Model file for the job. Use its own axes, mm. A direction names the side the tool comes from. Round coordinates to 2 decimals unless told otherwise and drop trailing zeros. Loops run counter-clockwise (first coordinate to the right, second up) from the corner with the lowest first, then second, coordinate; pieces in that order, holes last. Notation, with made-up numbers: M 40.5,-33.75 L 86.5,-33.75 A25 cw 86.5,3.25 Z; hole C 68,15 d5. An arc over 180 degrees is marked long. Use a Markdown table: item, result. Add a question column.
Item 1: Tool access for faces 1 (the flat face through (120, 300, -252)), 2 (the flat face through (120, 302.54, -252)), 3 (the cylindrical face through (103.313, 298.748, -38.394)): list every direction of +Z, -Z, +X, -X, +Y, -Y with a clear straight run to the whole face (end or side of a thin tool).
Item 2: Saw through at C-C on z = -101. Write the cut outline in (x, y), then the cut area to 3 significant figures.
Item 3: Saw through at A-A on y = 309. Write the cut outline in (x, z).
Item 4: Pin check, flat tips, straight feed: P1, Ø16.5, axis at x = 246, y = 314, coming from the -Z side; P2, Ø24.5, axis at x = 225.5, y = 320.5, coming from the +Z side; P3, Ø16.5, axis at y = 324.5, z = -182.5, coming from the +X side. Stop position of each tip, or through.
Item 5: Saw through at B-B on x = 30.5. Write the cut outline in (y, z).
Item 6: Saw through at D-D on z = -146. Write the cut outline in (x, y), then the cut area to 3 significant figures.
Item 7: Wall check: L1, parallel to Z at x = 194, y = 215; L2, parallel to X at y = 152, z = -27; L3, parallel to Y at x = 249.5, z = -224.5. Give the ranges that are in metal, low to high. Write a range as from..to.
Item 8: Two-plate mould, pull along X, no slides. Class faces 4 (the flat face through (148, 148, -300)), 5 (the flat face through (274.589, 316, -134)), 6 (the flat face through (148, 148, -297.46)): +X half, -X half, draft (parallel to the pull), parting line (faces both ways), or undercut.
```python
from build123d import *

# Parameters (mm, degrees)
SKETCH1_W           = 300
SKETCH1_H           = 300
BOSS_EXTRUDE1_DEPTH = 300
SHELL1_T            = -2.54
SKETCH2_W           = 300
SKETCH2_H           = 300
BOSS_EXTRUDE2_DEPTH = 2.54
SKETCH3_R           = 15.897271206
SKETCH3_R_2         = 16.201962057
SKETCH3_R_3         = 17.191821314
SKETCH3_R_4         = 17.661116969
CUT_EXTRUDE1_DEPTH  = 2.54
SKETCH4_R           = 22.06299853
SKETCH4_R_2         = 19.946075444
BOSS_EXTRUDE3_DEPTH = 2.54
SKETCH5_R           = 19.013382907
CUT_EXTRUDE2_DEPTH  = 2.54
SKETCH6_W           = 69.704124702
SKETCH6_H           = 204.3475123
SKETCH6_W_2         = 60.465312628
SKETCH6_H_2         = 192.466149128
BOSS_EXTRUDE4_DEPTH = 30.48
SKETCH7_W           = 69.704124702
SKETCH7_H           = 204.3475123
BOSS_EXTRUDE5_DEPTH = 2.54


with BuildPart() as part:
    # Sketch1 → Boss-Extrude1 (new body)
    with BuildSketch(Plane(origin=(0, 0, 0), x_dir=(1, 0, 0), z_dir=(0, 1, 0))):
        with Locations((150, 150)):
            Rectangle(SKETCH1_W, SKETCH1_H)
    extrude(amount=BOSS_EXTRUDE1_DEPTH)

    # Shell1
    shell1_openings = [part.faces().sort_by_distance(p)[0] for p in [
        (150, 300, -150),
    ]]
    offset(amount=SHELL1_T, openings=shell1_openings, kind=Kind.INTERSECTION)

    # Sketch2 → Boss-Extrude2 (add)
    with BuildSketch(Plane(origin=(0, 300, 0), x_dir=(1, 0, 0), z_dir=(0, 1, 0))):
        with Locations((150, 150)):
            Rectangle(SKETCH2_W, SKETCH2_H)
    extrude(amount=-BOSS_EXTRUDE2_DEPTH)

    # Sketch3 → Cut-Extrude1 (cut)
    with BuildSketch(Plane(origin=(0, 300, 0), x_dir=(1, 0, 0), z_dir=(0, 1, 0))):
        with Locations(Location((241.55793996, 57.94356866, 0), (0, 0, 270))):
            Circle(SKETCH3_R)
        with Locations(Location((241.55793996, 206.697112563, 0), (0, 0, 270))):
            Circle(SKETCH3_R_2)
        with Locations(Location((120.554438902, 251.95787292, 0), (0, 0, 270))):
            Circle(SKETCH3_R_3)
        with Locations(Location((120.554438902, 34.565752922, 0), (0, 0, 270))):
            Circle(SKETCH3_R_4)
    extrude(amount=-CUT_EXTRUDE1_DEPTH, mode=Mode.SUBTRACT)

    # Sketch4 → Boss-Extrude3 (add)
    with BuildSketch(Plane(origin=(0, 300, 0), x_dir=(1, 0, 0), z_dir=(0, 1, 0))):
        with Locations(Location((120.554438902, 251.95787292, 0), (0, 0, 90))):
            Circle(SKETCH4_R)
        with Locations(Location((241.55793996, 206.697112563, 0), (0, 0, 90))):
            Circle(SKETCH4_R_2)
    extrude(amount=BOSS_EXTRUDE3_DEPTH)

    # Sketch5 → Cut-Extrude2 (cut)
    with BuildSketch(Plane(origin=(0, 300, 0), x_dir=(1, 0, 0), z_dir=(0, 1, 0))):
        with Locations(Location((241.852973127, 150.869372117, 0), (0, 0, 270))):
            Circle(SKETCH5_R)
    extrude(amount=-CUT_EXTRUDE2_DEPTH, mode=Mode.SUBTRACT)

    # Sketch6 → Boss-Extrude4 (add)
    with BuildSketch(Plane(origin=(0, 300, 0), x_dir=(1, 0, 0), z_dir=(0, 1, 0))):
        with Locations((239.736552446, 135.332520717)):
            Rectangle(SKETCH6_W, SKETCH6_H)
        with Locations((239.510491416, 134.641215144)):
            Rectangle(SKETCH6_W_2, SKETCH6_H_2, mode=Mode.SUBTRACT)
    extrude(amount=BOSS_EXTRUDE4_DEPTH)

    # Sketch7 → Boss-Extrude5 (add)
    with BuildSketch(Plane(origin=(0, 330.48, 0), x_dir=(1, 0, 0), z_dir=(0, 1, 0))):
        with Locations((239.736552446, 135.332520717)):
            Rectangle(SKETCH7_W, SKETCH7_H)
    extrude(amount=BOSS_EXTRUDE5_DEPTH)


solid = part.part
```
Entries:
| question | item | result |
|---|---|---|
| 1 | face 1 | none |
| 1 | face 2 | +Z, -Z, -X, +Y |
| 1 | face 3 | +Y |
| 2 | outline | M 0,0 L 300,0 L 300,300 L 274.59,300 L 274.59,333.02 L 204.88,333.02 L 204.88,300 L 0,300 Z; hole M 2.54,2.54 L 297.46,2.54 L 297.46,297.46 L 2.54,297.46 Z; hole M 209.28,300 L 269.74,300 L 269.74,330.48 L 209.28,330.48 Z |
| 2 | area | 3,480 mm2 |
| 3 | outline | M 204.88,-237.51 L 274.59,-237.51 L 274.59,-33.16 L 204.88,-33.16 Z; hole M 209.28,-230.87 L 269.74,-230.87 L 269.74,-38.41 L 209.28,-38.41 Z |
| 4 | P1 | z = -237.51 |
| 4 | P2 | z = -33.16 |
| 4 | P3 | x = 274.59 |
| 5 | outline | M 0,-300 L 300,-300 L 300,0 L 0,0 Z; hole M 2.54,-297.46 L 297.46,-297.46 L 297.46,-2.54 L 2.54,-2.54 Z |
| 6 | outline | M 0,0 L 300,0 L 300,300 L 274.59,300 L 274.59,333.02 L 204.88,333.02 L 204.88,300 L 0,300 Z; hole M 2.54,2.54 L 297.46,2.54 L 297.46,297.46 L 260.23,297.46 L 260.23,300 L 269.74,300 L 269.74,330.48 L 209.28,330.48 L 209.28,300 L 223.47,300 L 223.47,297.46 L 2.54,297.46 Z |
| 6 | area | 3,390 mm2 |
| 7 | L1 | -300..-297.46, -2.54..0 |
| 7 | L2 | 0..2.54, 297.46..300 |
| 7 | L3 | 0..2.54, 297.46..302.54, 330.48..333.02 |
| 8 | face 4 | draft |
| 8 | face 5 | +X half |
| 8 | face 6 | undercut |
